Verification items for this drawing (mm, ordinates from the low corner). A direction names the side the tool comes from. Give positions to 0.01 mm unless a question says otherwise; leave off trailing zeros. Order: outer loops, then holes, each group sorted by start corner. A loop starts at its lowest first (then second) coordinate and runs counter-clockwise, first axis right, second up.
(1) Sectioned sample at A-A on x = 46. Record the cut outline in (y, z), plus the area to 3 significant figures.
(2) Access from +Z, -Z, +X, -X, +Y, -Y to the whole of each face (thin tool, end or side, straight path). Record for the marked faces 1, 2 and 3.
(3) Sectioned sample at C-C on z = 34.5. Record the cut outline in (x, y), plus the area to 3 significant figures.
(4) Scan lines: L1, parallel to Z at x = 16, y = 19; L2, parallel to X at y = 5.5, z = 36; L3, parallel to Y at x = 21.5, z = 27. Record each from-to range of solid material in increasing order.
(5) Gauge pin test, flat ends, axial feed: pin 1 (5 mm diameter, centred on x = 27.5, y = 14.5, fed in from +Z); pin 2 (8 mm diameter, centred on y = 8.5, z = 34, fed in from +X); pin 3 (8 mm diameter, centred on x = 40.5, y = 7.5, fed in from +Z). Record the tip position at first contact, or that the pin passes through.
(6) Sectioned sample at D-D on y = 11.5. Record the cut outline in (x, z), plus the area to 3 significant figures.
(7) Sectioned sample at B-B on y = 8. Record the cut outline in (x, z), plus the area to 4 significant figures.
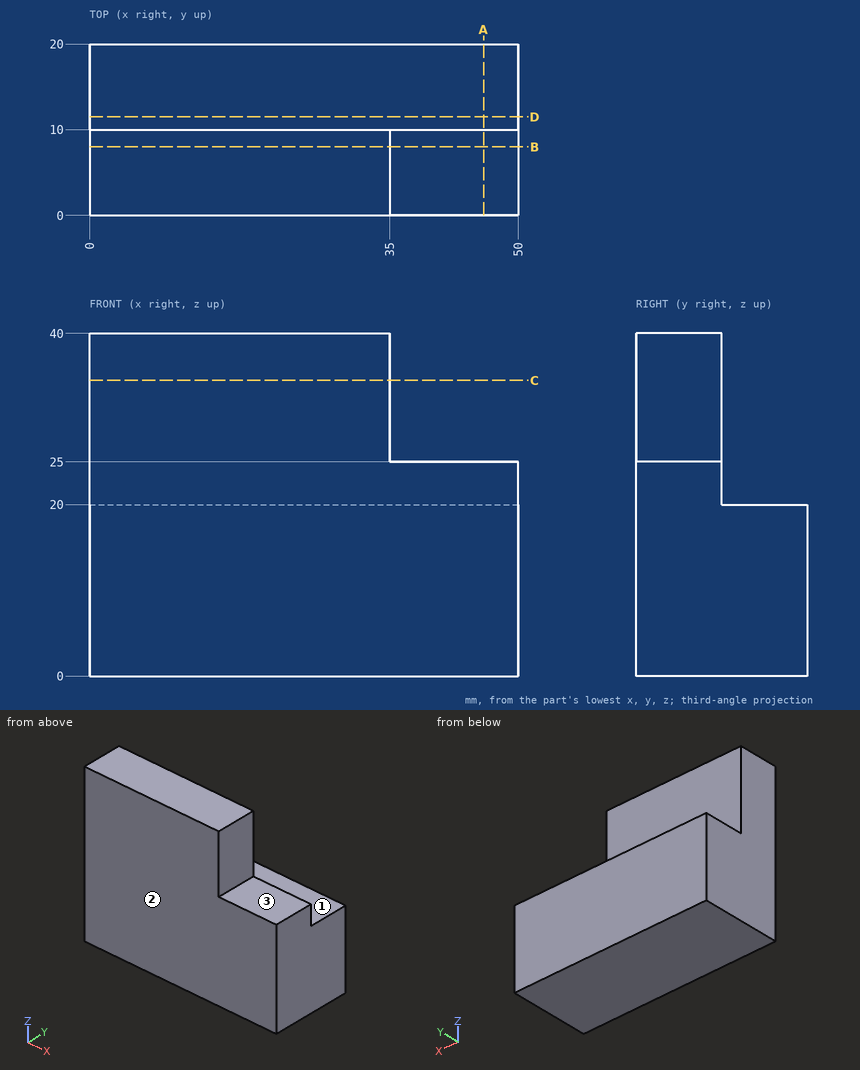
Ans:
1. outline: (0, 0) - (20, 0) - (20, 20) - (10, 20) - (10, 25) - (0, 25) - close
1. area: 450 mm2
2. face 1: +Z, +X, -X, +Y
2. face 2: +Z, -Z, +X, -X, -Y
2. face 3: +Z, +X, +Y, -Y
3. outline: (0, 0) - (35, 0) - (35, 10) - (0, 10) - close
3. area: 350 mm2
4. L1: z = 0 to 20
4. L2: x = 0 to 35
4. L3: y = 0 to 10
5. pin 1: stops at z = 20
5. pin 2: stops at x = 35
5. pin 3: stops at z = 25
6. outline: (0, 0) - (50, 0) - (50, 20) - (0, 20) - close
6. area: 1,000 mm2
7. outline: (0, 0) - (50, 0) - (50, 25) - (35, 25) - (35, 40) - (0, 40) - close
7. area: 1,775 mm2
